Work out the finished part from the listing and answer in its coordinate system (mm). Face numbers are marked on the shaded views. A direction names the side the tool comes from. Coordinates: 2 decimals unless noted, no trailing zeros. Write each loop counter-clockwise with the first axis right and the second up, starting at its lowest first coordinate (ties: lowest second). Pieces come first, ordered by that corner, then holes. Notation, with made-up numbers: (31.25, 45) - (51.25, 45) arc R25 ccw to (51.25, 73) - close; hole circle Ø1 at (53, 69.25). An arc over 180 degrees is marked (long way). Use a Markdown table: item, result. Add a question column.
(1) The part is cut by section D-D, the plane y = 16. Give the vertices of the cut face in (x, z).
(2) Given pin 1 Ø5.5 at (x, y) = (15, 15) entering from -Z; pin 2 Ø12 at (x, y) = (12.5, 7) entering from +Z; pin 3 Ø8 at (x, y) = (13, 10) entering from +Z; pin 4 Ø3 at (x, z) = (7.5, 20.5) entering from -Y, each flat-ended and moving along its own axis, determine where each tip first touches the part or whether it passes through.
(3) Find the intervals of material crossed by line 1 (Y direction, x = 15, z = 0.85); line 2 (Y direction, x = 15, z = 9); line 3 (Y direction, x = 14.75, z = 18), in increasing order. Write a range as from..to.
(4) A tool of negligible diameter and unlimited length cuts with its end or side. For the marked faces 1, 2 and 3, from which of +Z, -Z, +X, -X, +Y, -Y can it reach the whole face along a straight path? Write none if from no direction.
(5) For a pull along Y with two mould halves and no side action, classify the marked faces 4, 5 and 6 as released by +Y, released by -Y, zero draft, split by the parting line, or undercut.
(6) The part is cut by section C-C, the plane x = 7.5. Give the vertices of the cut face in (y, z), then the cut area to 3 significant figures.
(7) The part is cut by section A-A, the plane z = 18.5. Give the vertices of the cut face in (x, y).
(8) The part is cut by section B-B, the plane y = 35. Give the vertices of the cut face in (x, z).
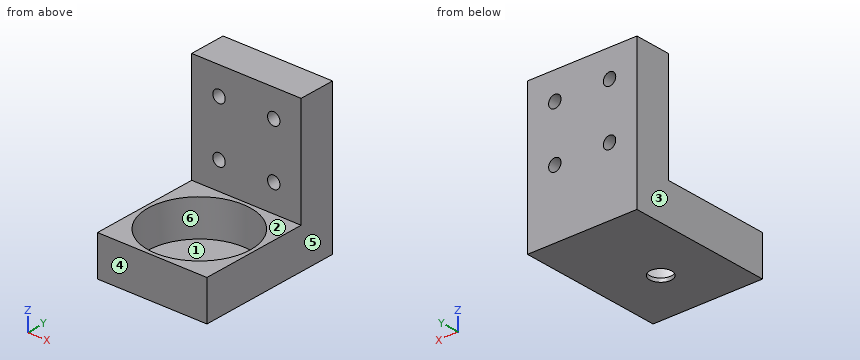
from build123d import *

# Parameters (mm, degrees)
SKETCH1_W           = 30
SKETCH1_H           = 30
BOSS_EXTRUDE1_DEPTH = 11
SKETCH2_R           = 14
CUT_EXTRUDE1_DEPTH  = 10
SKETCH3_R           = 3
CUT_EXTRUDE2_DEPTH  = 1
SKETCH4_W           = 30
SKETCH4_H           = 41
BOSS_EXTRUDE2_DEPTH = 10
SKETCH5_R           = 1.7
CUT_EXTRUDE3_DEPTH  = 60


with BuildPart() as part:
    # Sketch1 → Boss-Extrude1 (new body)
    with BuildSketch(Plane.XY):
        with Locations((15, 15)):
            Rectangle(SKETCH1_W, SKETCH1_H)
    extrude(amount=BOSS_EXTRUDE1_DEPTH)

    # Sketch2 → Cut-Extrude1 (cut)
    with BuildSketch(Plane.XY.offset(11)):
        with Locations((15, 15)):
            Circle(SKETCH2_R)
    extrude(amount=-CUT_EXTRUDE1_DEPTH, mode=Mode.SUBTRACT)

    # Sketch3 → Cut-Extrude2 (cut)
    with BuildSketch(Plane.XY.offset(1)):
        with Locations((15, 15)):
            Circle(SKETCH3_R)
    extrude(amount=-CUT_EXTRUDE2_DEPTH, mode=Mode.SUBTRACT)

    # Sketch4 → Boss-Extrude2 (add)
    with BuildSketch(Plane(origin=(0, 30, 0), x_dir=(1, 0, 0), z_dir=(0, 1, 0))):
        with Locations((15, -20.5)):
            Rectangle(SKETCH4_W, SKETCH4_H)
    extrude(amount=BOSS_EXTRUDE2_DEPTH)

    # Sketch5 → Cut-Extrude3 (cut, through all)
    with BuildSketch(Plane.XZ.offset(-30)):
        with Locations(Location((7.5, 33.5, 0), (0, 0, 270))):
            Circle(SKETCH5_R)
        with Locations(Location((22.5, 33.5, 0), (0, 0, 270))):
            Circle(SKETCH5_R)
        with Locations(Location((7.5, 18.5, 0), (0, 0, 270))):
            Circle(SKETCH5_R)
        with Locations(Location((22.5, 18.5, 0), (0, 0, 270))):
            Circle(SKETCH5_R)
    extrude(amount=-CUT_EXTRUDE3_DEPTH, mode=Mode.SUBTRACT)


solid = part.part
Model answer:
| question | item | result |
|---|---|---|
| 1 | outline | (0, 0) - (12.17, 0) - (12.17, 1) - (1.04, 1) - (1.04, 11) - (0, 11) - close; (17.83, 0) - (30, 0) - (30, 11) - (28.96, 11) - (28.96, 1) - (17.83, 1) - close |
| 2 | pin 1 | through |
| 2 | pin 2 | z = 11 |
| 2 | pin 3 | z = 1 |
| 2 | pin 4 | y = 30 |
| 3 | line 1 | 0..12, 18..40 |
| 3 | line 2 | 0..1, 29..40 |
| 3 | line 3 | 30..40 |
| 4 | face 1 | +Z |
| 4 | face 2 | +Z, +X, -X, -Y |
| 4 | face 3 | +Z, -Z, -X, +Y, -Y |
| 5 | face 4 | released by -Y |
| 5 | face 5 | zero draft |
| 5 | face 6 | undercut |
| 6 | outline | (0, 0) - (40, 0) - (40, 16.8) - (30, 16.8) - (30, 11) - (26.82, 11) - (26.82, 1) - (3.18, 1) - (3.18, 11) - (0, 11) - close; (30, 20.2) - (40, 20.2) - (40, 31.8) - (30, 31.8) - close; (30, 35.2) - (40, 35.2) - (40, 41) - (30, 41) - close |
| 6 | area | 436 mm^2 |
| 7 | outline | (0, 30) - (5.8, 30) - (5.8, 40) - (0, 40) - close; (9.2, 30) - (20.8, 30) - (20.8, 40) - (9.2, 40) - close; (24.2, 30) - (30, 30) - (30, 40) - (24.2, 40) - close |
| 8 | outline | (0, 0) - (30, 0) - (30, 41) - (0, 41) - close; hole circle Ø3.4 at (7.5, 18.5); hole circle Ø3.4 at (7.5, 33.5); hole circle Ø3.4 at (22.5, 18.5); hole circle Ø3.4 at (22.5, 33.5) |
